```python
from build123d import *

# Parameters (mm, degrees)
FILLET1_R = 1.524
FILLET2_R = 0.508


with BuildPart() as part:
    # Sketch3 → Revolve1 (revolve)
    with BuildSketch(Plane(origin=(0, 0, 0), x_dir=(0, 0, -1), z_dir=(1, 0, 0))):
        Polygon((-12.813309339, -42.7101), (50.6476, -42.7101), (50.6476, -36.6903), (2.3876, -36.6903), (2.3876, -34.798), (-2.3876, -34.798), (-2.3876, -36.6903), (-50.6476, -36.6903), (-50.6476, -42.0497), align=None)
    revolve(axis=Axis((0, 0, 50.6476), (0, 0, -1)))

    # Fillet1
    fillet1_edges = [part.edges().sort_by_distance(p)[0] for p in [
        (0, 36.6903, -50.6476),
        (0, 36.6903, 50.6476),
    ]]
    fillet(fillet1_edges, radius=FILLET1_R)

    # Fillet2
    fillet2_edges = [part.edges().sort_by_distance(p)[0] for p in [
        (0, 36.6903, 2.3876),
        (0, 36.6903, -2.3876),
    ]]
    fillet(fillet2_edges, radius=FILLET2_R)


solid = part.part
```
Check sheet for the modelled part. Datum: model origin and axes. Units: mm. A direction names the side the tool comes from. Round coordinates to 2 decimals unless told otherwise and drop trailing zeros. Order: outer loops, then holes, each group sorted by start corner. A loop starts at its lowest first (then second) coordinate and runs counter-clockwise, first axis right, second up. Notation, with made-up numbers: (64.25, 54) -> (108.25, 54) arc R35 ccw to (108.25, 92) -> close; hole circle Ø10 at (30.5, 38.5). An arc over 180 degrees is marked (long way). One line per item, written item: value. Start each with the question number.
Q1. Thickness scan on line 1 (Y direction, x = 0, z = -28.5); line 2 (X direction, y = 0, z = 0.65). Record the ranges inside material, lowest first.
Q2. Cross-section at A-A (z = 9.5). Record the boundary of the cut face in (x, y), and give its area (3 significant figures).
Q3. Set-up check for faces 4 (the face through (-36.378, 4.776, 26.333)), 5 (the face through (-36.378, 4.776, -25.686)), 6 (the face through (-12.829, -40.738, -19.361)): record each of +Z, -Z, +X, -X, +Y, -Y from which the full face is reachable in a straight line by a thin tool's end or side.
Q4. Cross-section at B-B (z = 29.5). Record the boundary of the cut face in (x, y).
Q5. Gauge pin test, flat ends, axial feed: pin 1 Ø1 at (y, z) = (-8, -30) entering from -X; pin 2 Ø10 at (x, z) = (-24.5, 11) entering from -Y. Record the tip position at first contact, or that the pin passes through.
Q6. Mould release check, pull along Y, two halves, no side actions. Record for faces 1 (the face through (22, 32, -50.648)), 2 (the face through (-30, -19, 2.388)), 3 (the face through (25.79, 33.635, 31.466)): pulls with the +Y half, pulls with the -Y half, needs draft (parallel to the pull), parting line crosses it, or undercut.
Completed:
1. line 1: y = -42.71 to -36.69, 36.69 to 42.71
1. line 2: x = -42.71 to -34.8, 34.8 to 42.71
2. outline: circle Ø85.42 at (0, 0); hole circle Ø73.38 at (0, 0)
2. area: 1,500 mm²
3. face 4: +Z
3. face 5: -Z
3. face 6: +Z, -Z
4. outline: circle Ø84.84 at (0, 0); hole circle Ø73.38 at (0, 0)
5. pin 1: stops at x = -42.05
5. pin 2: stops at y = -38
6. face 1: needs draft
6. face 2: undercut
6. face 3: parting line crosses it
